```python
from build123d import *

# Parameters (mm, degrees)
BOSS_EXTRUDE1_DEPTH    = 5.08
F_10_CLEARANCE_HOLE1_D = 4.9784


with BuildPart() as part:
    # Sketch1 → Boss-Extrude1 (new body)
    with BuildSketch(Plane(origin=(0, 0, 0), x_dir=(1, 0, 0), z_dir=(0, 1, 0))):
        with BuildLine():
            Line((27.234807671, -40.223012788), (-5.482691703, -74.830900036))
            ThreePointArc((-5.482691703, -74.830900036), (-11.874952903, -74.014978741), (-13.943081074, -67.911735613))
            Line((-13.943081074, -67.911735613), (29.080561657, -3.550446088))
            Line((29.080561657, -3.550446088), (77.831071682, -3.550446088))
            Line((77.831071682, -3.550446088), (77.831071682, -39.427946088))
            Line((77.831071682, -39.427946088), (29.080561657, -39.427946088))
            ThreePointArc((29.080561657, -39.427946088), (28.075706091, -39.635165496), (27.234807671, -40.223012788))
        make_face()
    extrude(amount=BOSS_EXTRUDE1_DEPTH)

    # #10 Clearance Hole1 (through all)
    with Locations(Plane(origin=(0, 5.08, 0), x_dir=(1, 0, 0), z_dir=(0, 1, 0))):
        with Locations((42.63541667, -33.427196088), (42.63541667, -9.551196088), (64.27621667, -9.551196088), (64.27621667, -33.427196088)):
            Hole(F_10_CLEARANCE_HOLE1_D / 2)


solid = part.part
```
Part model, mm, in its own coordinate system. A direction names the side the tool comes from. Round coordinates to 2 decimals unless told otherwise and drop trailing zeros. Loops run counter-clockwise (first coordinate to the right, second up) from the corner with the lowest first, then second, coordinate; pieces in that order, holes last. Notation, with made-up numbers: (46.25, 38) -> (83.25, 38) arc R28 cw to (83.25, 58) -> close; hole circle Ø9 at (43.25, 12). An arc over 180 degrees is marked (long way). Use one line per item in the form item = value. Start each with the question number.
Item 1: Drop a flat-ended pin along its axis: pin 1 Ø3 at (y, z) = (2.5, 41) entering from -X. Give the stop position or say it passes through.
Item 2: Tool access for faces 4 (the flat face through (54, 3, 39.428)), 5 (the cylindrical face through (61.977, 2.504, 34.381)): list every direction of +Z, -Z, +X, -X, +Y, -Y with a clear straight run to the whole face (end or side of a thin tool).
Item 3: Band-saw the part on A-A (x = 44). List the corners of the cut face in (y, z).
Item 4: Band-saw the part on B-B (z = 32). List the corners of the cut face in (x, y).
Item 5: Band-saw the part on C-C (y = 0.9). List the corners of the cut face in (x, z), plus the area to 3 significant figures.
Item 6: Drill centre lines: line 1 along Z through (x, y) = (66, 3.05); line 2 along X through (y, z) = (0.2, 11.5); line 3 along X through (y, z) = (4.4, 33). Where is each one in solid material? Low to high.
Item 7: Two-plate mould, pull along Z, no slides. Class faces 1 (the flat face through (77.831, 3, 21)), 2 (the flat face through (53, 3, 3.55)), 3 (the cylindrical face through (61.977, 2.504, 10.505)): released by +Z, released by -Z, zero draft, split by the parting line, or undercut.
Item 8: Band-saw the part on D-D (x = 57). List the corners of the cut face in (y, z).
Data:
q1.pin_1 = 3.04
q2.face_4 = +Z, +X, +Y, -Y
q2.face_5 = +Y, -Y
q3.outline = (0, 3.55) -> (5.08, 3.55) -> (5.08, 7.47) -> (0, 7.47) -> close; (0, 11.63) -> (5.08, 11.63) -> (5.08, 31.35) -> (0, 31.35) -> close; (0, 35.51) -> (5.08, 35.51) -> (5.08, 39.43) -> (0, 39.43) -> close
q4.outline = (10.06, 0) -> (40.6, 0) -> (40.6, 5.08) -> (10.06, 5.08) -> close; (44.67, 0) -> (62.24, 0) -> (62.24, 5.08) -> (44.67, 5.08) -> close; (66.32, 0) -> (77.83, 0) -> (77.83, 5.08) -> (66.32, 5.08) -> close
q5.outline = (-13.94, 67.91) -> (29.08, 3.55) -> (77.83, 3.55) -> (77.83, 39.43) -> (29.08, 39.43) arc R2.54 cw to (27.23, 40.22) -> (-5.48, 74.83) arc R6.08 ccw to start; hole circle Ø4.98 at (42.64, 9.55); hole circle Ø4.98 at (42.64, 33.43); hole circle Ø4.98 at (64.28, 9.55); hole circle Ø4.98 at (64.28, 33.43)
q5.area = 2,720 mm^2
q6.line_1 = 3.55 to 7.76, 11.35 to 31.63, 35.22 to 39.43
q6.line_2 = 23.77 to 41.09, 44.18 to 62.73, 65.82 to 77.83
q6.line_3 = 9.39 to 40.18, 45.09 to 61.82, 66.73 to 77.83
q7.face_1 = zero draft
q7.face_2 = released by -Z
q7.face_3 = undercut
q8.outline = (0, 3.55) -> (5.08, 3.55) -> (5.08, 39.43) -> (0, 39.43) -> close
